Geometry: final body of the model. Coordinates: model frame, mm. A direction names the side the tool comes from. Give positions to 0.01 mm unless a question says otherwise; leave off trailing zeros. Write each loop counter-clockwise with the first axis right and the second up, starting at its lowest first coordinate (ties: lowest second). Pieces come first, ordered by that corner, then holes.
Q1. Cut plane A-A on x = 5.75. Return the cut outline in (y, z).
Q2. Cut plane C-C on z = 0. Return the cut outline in (x, y).
Q3. Pin query (flat end, axial travel): pin 1 (3.5 mm diameter, centred on y = 0.5, z = 1.5, fed in from +X); pin 2 (5 mm diameter, centred on x = 0, z = 40, fed in from -Y); pin 3 (10 mm diameter, centred on x = 1.5, z = 55.5, fed in from -Y). Return the tip coordinate at first contact, or that it passes through.
Q4. Cut plane D-D on x = -0.75. Return the cut outline in (y, z).
Q5. Reachability of faces 1 (the face through (6, -3.5, 0)), 2 (the face through (6, 3.5, 0)), 3 (the face through (3, -2, 3.5)) from +Z, -Z, +X, -X, +Y, -Y: full face, straight path, thin tool, end or side. Return the list, or none.
Q6. Cut plane B-B on y = 0. Return the cut outline in (x, z), plus the area to 4 significant figures.
Q7. Draft query along Z for faces 4 (the face through (6, 0, -3.5)), 5 (the face through (1, 0, 3)), 6 (the face through (1.78, -3.04, 42.15)), 7 (the face through (8.52, -1.15, 4.98)). Return one class per face: pulls with the +Z half, pulls with the -Z half, needs draft (parallel to the pull), parting line crosses it, or undercut.
Q8. Line query: L1, parallel to Z at x = 9.25, y = -0.25; L2, parallel to X at y = 0.25, z = 48.5; L3, parallel to Z at x = 8, y = 3.75. Output: solid intervals per line, ascending.
```python
from build123d import *

# Parameters (mm, degrees)
SKETCH1_R              = 5
BARREL_CONNECTOR_DEPTH = 8.5
SKETCH2_R              = 3
BOSS_EXTRUDE2_DEPTH    = 2
SKETCH3_W              = 7
SKETCH3_H              = 7
BOSS_EXTRUDE3_DEPTH    = 7.5
SKETCH4_R              = 3
BOSS_EXTRUDE4_DEPTH    = 3
SKETCH5_R              = 5.5
BOSS_EXTRUDE5_DEPTH    = 11
SKETCH6_R              = 5
BOSS_EXTRUDE6_DEPTH    = 50


with BuildPart() as part:
    # Sketch1 → Barrel Connector (new body)
    with BuildSketch(Plane(origin=(0, 0, 0), x_dir=(0, 0, -1), z_dir=(1, 0, 0))):
        Circle(SKETCH1_R)
    extrude(amount=-BARREL_CONNECTOR_DEPTH)

    # Sketch2 → Boss-Extrude2 (add)
    with BuildSketch(Plane(origin=(0, 0, 0), x_dir=(0, 0, -1), z_dir=(1, 0, 0))):
        Circle(SKETCH2_R)
    extrude(amount=BOSS_EXTRUDE2_DEPTH)

    # Sketch3 → Boss-Extrude3 (add)
    with BuildSketch(Plane(origin=(2, 0, 0), x_dir=(0, 0, -1), z_dir=(1, 0, 0))):
        Rectangle(SKETCH3_W, SKETCH3_H)
    extrude(amount=BOSS_EXTRUDE3_DEPTH)

    # Sketch4 → Boss-Extrude4 (add)
    with BuildSketch(Plane.XY.offset(3.5)):
        with Locations((5.75, 0)):
            Circle(SKETCH4_R)
    extrude(amount=BOSS_EXTRUDE4_DEPTH)

    # Sketch5 → Boss-Extrude5 (add)
    with BuildSketch(Plane.XY.offset(6.5)):
        with Locations((5.75, 0)):
            Circle(SKETCH5_R)
    extrude(amount=BOSS_EXTRUDE5_DEPTH)

    # Sketch6 → Boss-Extrude6 (add)
    with BuildSketch(Plane.XY.offset(17.5)):
        with Locations((5.75, 0)):
            Circle(SKETCH6_R)
    extrude(amount=BOSS_EXTRUDE6_DEPTH)


solid = part.part
```
Data:
1. outline: (-5.5, 6.5) - (-3, 6.5) - (-3, 3.5) - (-3.5, 3.5) - (-3.5, -3.5) - (3.5, -3.5) - (3.5, 3.5) - (3, 3.5) - (3, 6.5) - (5.5, 6.5) - (5.5, 17.5) - (5, 17.5) - (5, 67.5) - (-5, 67.5) - (-5, 17.5) - (-5.5, 17.5) - close
2. outline: (-8.5, -5) - (0, -5) - (0, -3) - (2, -3) - (2, -3.5) - (9.5, -3.5) - (9.5, 3.5) - (2, 3.5) - (2, 3) - (0, 3) - (0, 5) - (-8.5, 5) - close
3. pin 1: stops at x = 9.5
3. pin 2: stops at y = -3.8
3. pin 3: stops at y = -5
4. outline: circle Ø10 at (0, 0)
5. face 1: -Z, +X, -Y
5. face 2: -Z, +X, +Y
5. face 3: none
6. outline: (-8.5, -5) - (0, -5) - (0, -3) - (2, -3) - (2, -3.5) - (9.5, -3.5) - (9.5, 3.5) - (8.75, 3.5) - (8.75, 6.5) - (11.25, 6.5) - (11.25, 17.5) - (10.75, 17.5) - (10.75, 67.5) - (0.75, 67.5) - (0.75, 17.5) - (0.25, 17.5) - (0.25, 6.5) - (2.75, 6.5) - (2.75, 3.5) - (2, 3.5) - (2, 3) - (0, 3) - (0, 5) - (-8.5, 5) - close
6. area: 788.5 mm2
7. face 4: pulls with the -Z half
7. face 5: undercut
7. face 6: needs draft
7. face 7: undercut
8. L1: z = -3.5 to 3.5, 6.5 to 67.5
8. L2: x = 0.76 to 10.74
8. L3: z = 6.5 to 67.5
